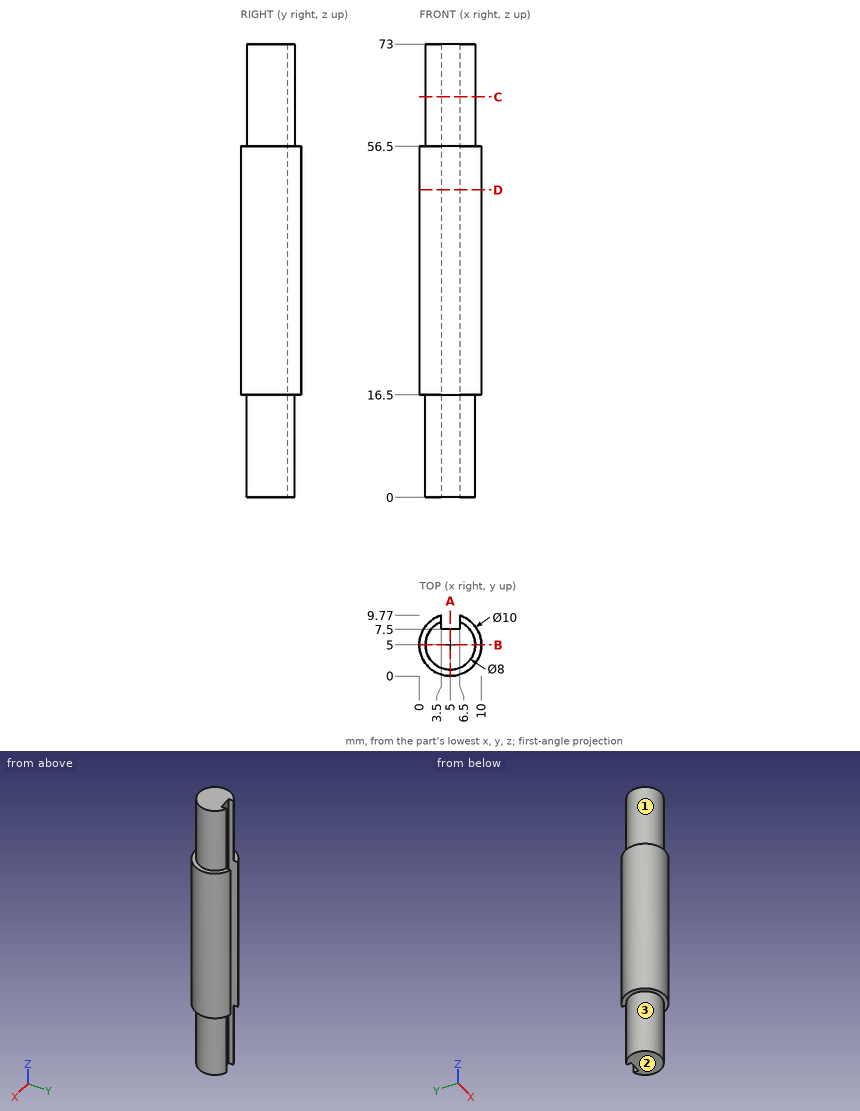
Print and shaded views of the part. All mm, measured from the part's lowest x, y and z. A direction names the side the tool comes from. Coordinates: 2 decimals unless noted, no trailing zeros. Loops run counter-clockwise (first coordinate to the right, second up) from the corner with the lowest first, then second, coordinate; pieces in that order, holes last. Notation, with made-up numbers: (70.25, 61) -> (83.25, 61) arc R24 cw to (83.25, 78) -> close; hole circle Ø10 at (85, -39). An arc over 180 degrees is marked (long way). Use one line per item in the form item = value. Start each with the question number.
(1) Probe probe 1 along X at (y, z) = (7.75, 66) (1 decimal); probe 2 along Y at (x, z) = (5, 22); probe 3 along Y at (x, z) = (7.25, 55.5) (1 decimal). List the from-to ranges inside material, lowest first. Write a range as from..to.
(2) Flat gauge pins, fed straight in: pin 1 (1 mm diameter, centred on y = 8.5, z = 17.5, fed in from +X); pin 2 (2.5 mm diameter, centred on x = 4.5, z = 51, fed in from +Y); pin 3 (2.5 mm diameter, centred on y = 8, z = 46.5, fed in from +X); pin 4 (1.5 mm diameter, centred on x = 4, z = 25.5, fed in from -Y). Where does each tip first touch, or does it go through?
(3) Tool access for the marked faces 1, 2 and 3: list every direction of +Z, -Z, +X, -X, +Y, -Y with a clear straight run to the whole face (end or side of a thin tool).
(4) Cut at D-D on z = 49.5. Give the cut face in (x, y).
(5) Cut at C-C on z = 64.5. Give the cut face in (x, y).
(6) Cut at A-A on x = 5. Give the cut face in (y, z).
(7) Cut at B-B on y = 5. Give the cut face in (x, z), and give its area (3 significant figures).
Values:
q1.probe_1 = 2.1..3.5, 6.5..7.9
q1.probe_2 = 0..7.5
q1.probe_3 = 0.5..9.5
q2.pin_1 = 9
q2.pin_2 = 9.77
q2.pin_3 = 9.68
q2.pin_4 = 0.01
q3.face_1 = +Z
q3.face_2 = -Z, +X, -X, +Y, -Y
q3.face_3 = -Z
q4.outline = (3.5, 7.5) -> (3.5, 9.77) arc R5 ccw (long way) to (6.5, 9.77) -> (6.5, 7.5) -> close
q5.outline = (3.5, 7.5) -> (3.5, 8.71) arc R4 ccw (long way) to (6.5, 8.71) -> (6.5, 7.5) -> close
q6.outline = (0, 16.5) -> (1, 16.5) -> (1, 0) -> (7.5, 0) -> (7.5, 73) -> (1, 73) -> (1, 56.5) -> (0, 56.5) -> close
q7.outline = (0, 16.5) -> (1, 16.5) -> (1, 0) -> (9, 0) -> (9, 16.5) -> (10, 16.5) -> (10, 56.5) -> (9, 56.5) -> (9, 73) -> (1, 73) -> (1, 56.5) -> (0, 56.5) -> close
q7.area = 664 mm2
